The figure shows three views and two pictorial views of one solid part (mm, origin at its lowest corner). Answer the questions. A direction names the side the tool comes from. Coordinates: 2 decimals unless noted, no trailing zeros. Loops run counter-clockwise (first coordinate to the right, second up) from the corner with the lowest first, then second, coordinate; pieces in that order, holes last. Notation, with made-up numbers: M 33,-38.5 L 61,-38.5 A19 cw 61,-11.5 Z; hole C -27.5,84 d4. An arc over 180 degrees is marked long. Write each question's results on one line, items separated by ' | '.
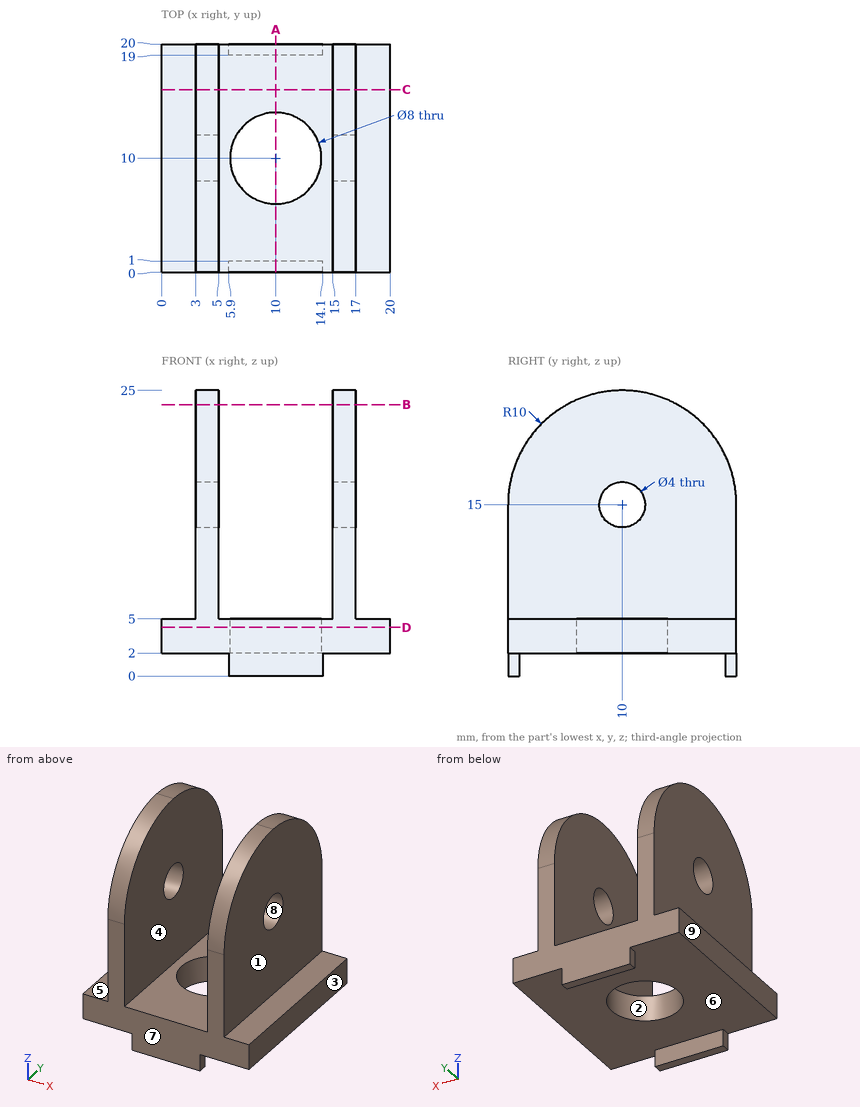
1) For a pull along Y with two mould halves and no side action, classify the marked faces 6, 7, 8 and 9 as released by +Y, released by -Y, zero draft, split by the parting line, or undercut.
Check result:
face 6: undercut | face 7: released by -Y | face 8: undercut | face 9: zero draft
2) Given pin 1 Ø1 at (x, y) = (15.5, 6.5) entering from -Z; pin 2 Ø3 at (x, y) = (10, 11.5) entering from -Z; pin 3 Ø6 at (x, y) = (10.5, 4.5) entering from +Z; pin 4 Ø1.1 at (y, z) = (0.5, 0.5) entering from +X, each flat-ended and moving along its own axis, determine where each tip first touches the part or whether it passes through.
Check result:
pin 1: z = 2 | pin 2: through | pin 3: z = 5 | pin 4: x = 14.1
3) Find section D-D, the plane z = 4.25. Give the vertices of the cut face in (x, y), and give its area (3 significant figures).
Check result:
outline: M 0,0 L 20,0 L 20,20 L 0,20 Z; hole C 10,10 d8 | area: 350 mm^2
4) Straight lines are drawn through the part: probe 1 along Y at (x, z) = (10, 4.15); probe 2 along X at (y, z) = (18.5, 19.25); probe 3 along Y at (x, z) = (15.5, 15). For each, find the intervals that lie inside material, in ascending order. Write a range as [from, to].
Check result:
probe 1: [0, 6], [14, 20] | probe 2: [3, 5], [15, 17] | probe 3: [0, 8], [12, 20]
5) Find section C-C, the plane y = 16. Give the vertices of the cut face in (x, z).
Check result:
outline: M 0,2 L 20,2 L 20,5 L 17,5 L 17,23 L 15,23 L 15,5 L 5,5 L 5,23 L 3,23 L 3,5 L 0,5 Z
6) Find section A-A, the plane x = 10. Give the vertices of the cut face in (y, z), and give its area (3 significant figures).
Check result:
outline: M 0,0 L 1,0 L 1,2 L 6,2 L 6,5 L 0,5 Z; M 14,2 L 19,2 L 19,0 L 20,0 L 20,5 L 14,5 Z | area: 40.0 mm^2
7) Which of the six approach directions +Z, -Z, +X, -X, +Y, -Y give full straight-line access (tool end or side, diameter ignored) to the marked faces 1, 2, 3, 4 and 5?
Check result:
face 1: +Z, +X, +Y, -Y | face 2: +Z, -Z | face 3: +Z, -Z, +X, +Y, -Y | face 4: +Z, +Y, -Y | face 5: +Z, -X, +Y, -Y
8) Find section B-B, the plane z = 23.75. Give the vertices of the cut face in (x, y).
Check result:
outline: M 3,5.16 L 5,5.16 L 5,14.84 L 3,14.84 Z; M 15,5.16 L 17,5.16 L 17,14.84 L 15,14.84 Z
